Part model, mm, in its own coordinate system. A direction names the side the tool comes from. Round coordinates to 2 decimals unless told otherwise and drop trailing zeros. Loops run counter-clockwise (first coordinate to the right, second up) from the corner with the lowest first, then second, coordinate; pieces in that order, holes last. Notation, with made-up numbers: M 44.5,-20.75 L 80.5,-20.75 A21 ccw 80.5,10.25 Z; hole C 83.5,-15.5 d5. An arc over 180 degrees is marked long. Put each result on its own line as item: value. Start each with the question number.
1) Slice it at A-A on x = 0. Give the cut face in (y, z).
2) Pull direction Z, two halves, no side cores. Call faces 6 (the flat face through (0, 0, -22.149)), 7 (the flat face through (9.112, 0, -11)), 8 (the cylindrical face through (-27.2, 0, -10.4)): +Z half, -Z half, draft (parallel to the pull), parting line (faces both ways), or undercut.
3) Drop flat-ended pins along their axis: pin 1 Ø6 at (y, z) = (0.5, -15.5) entering from -X; pin 2 Ø6 at (x, z) = (-32, -2) entering from +Y; pin 3 Ø1.5 at (x, z) = (-21, -12) entering from +Y; pin 4 Ø6 at (y, z) = (17.5, -3) entering from +X. Give the stop position or say it passes through.
4) Slice it at C-C on y = -19. Give the cut face in (x, z).
5) Slice it at B-B on z = -1. Give the cut face in (x, y).
6) Probe line 1 along X through (y, z) = (-7, 6); line 2 along X through (y, z) = (-5, 16); line 3 along Y through (x, z) = (-37.5, 21.9). List the from-to ranges inside material, lowest first.
7) Slice it at D-D on x = -17. Give the cut face in (y, z), then the cut area to 3 significant figures.
8) Which spindle directions (+Z, -Z, +X, -X, +Y, -Y) get a long thin tool onto all of the face, cutting with end or side? Do faces 1 (the flat face through (29, -2.75, -9)), 2 (the flat face through (0, 2.75, -9)), 3 (the cylindrical face through (-1.84, 14.04, 33.52)), 4 (the flat face through (20.098, 0, -11)), 5 (the flat face through (-38.322, 0, -11)). Say none if no direction does.
```python
from build123d import *

# Parameters (mm, degrees)
SKETCH1_R                = 14.1605
BOSS_EXTRUDE1_DEPTH      = 43.18
SKETCH3_W                = 18.2245
SKETCH3_H                = 22.1488
SKETCH3_R                = 4.2545
BOSS_EXTRUDE2_DEPTH      = 2.74955
BOSS_EXTRUDE2_DEPTH_BACK = 2.74955
LPATTERN1_COUNT          = 2
LPATTERN1_PITCH          = 29.21
LPATTERN1_2_COUNT        = 2
LPATTERN1_2_PITCH        = 29.21
BOSS_EXTRUDE3_START      = 20.32
SKETCH4_R                = 3.048
BOSS_EXTRUDE3_DEPTH      = 3.81
BOSS_EXTRUDE4_START      = -30.48
BOSS_EXTRUDE4_DEPTH      = 2.54


with BuildPart() as part:
    # Sketch1 → Boss-Extrude1 (new body)
    with BuildSketch(Plane.XY):
        Circle(SKETCH1_R)
    extrude(amount=BOSS_EXTRUDE1_DEPTH)

    # Sketch3 → Boss-Extrude2 (add, two sides)
    with BuildSketch(Plane(origin=(0, 0, 0), x_dir=(1, 0, 0), z_dir=(0, 1, 0))) as boss_extrude2_sk:
        with Locations((0, 11.0744)):
            Rectangle(SKETCH3_W, SKETCH3_H)
        with Locations((0, 14.1478)):
            Circle(SKETCH3_R, mode=Mode.SUBTRACT)
    extrude(amount=BOSS_EXTRUDE2_DEPTH)
    extrude(boss_extrude2_sk.sketch, amount=-BOSS_EXTRUDE2_DEPTH_BACK)


with BuildPart() as lpattern1_1:
    # LPattern1: pattern copy
    add(part.part.moved(Location(Vector(1, 0, 0) * (1 * LPATTERN1_PITCH))))


with BuildPart() as lpattern1_2_1:
    # LPattern1 2: pattern copy
    add(part.part.moved(Location(Vector(-1, 0, 0) * (1 * LPATTERN1_2_PITCH))))


with BuildPart() as lpattern1_2_2:
    # LPattern1 2: pattern copy
    add(lpattern1_1.part.moved(Location(Vector(-1, 0, 0) * (1 * LPATTERN1_2_PITCH))))


with BuildPart() as part_1:
    add(part.part)

    add(lpattern1_1.part)  # Boss-Extrude3 merges LPattern1_1

    add(lpattern1_2_1.part)  # Boss-Extrude3 merges LPattern1 2_1

    add(lpattern1_2_2.part)  # Boss-Extrude3 merges LPattern1 2_2
    # Sketch4 → Boss-Extrude3 (add)
    with BuildSketch(Plane.XY.offset(BOSS_EXTRUDE3_START)):
        with BuildLine():
            Line((-37.5, 24), (37.5, 24))
            ThreePointArc((37.5, 24), (44.571067812, 21.071067812), (47.5, 14))
            Line((47.5, 14), (47.5, -14))
            ThreePointArc((47.5, -14), (44.571067812, -21.071067812), (37.5, -24))
            Line((37.5, -24), (-37.5, -24))
            ThreePointArc((-37.5, -24), (-44.571067812, -21.071067812), (-47.5, -14))
            Line((-47.5, -14), (-47.5, 14))
            ThreePointArc((-47.5, 14), (-44.571067812, 21.071067812), (-37.5, 24))
        make_face()
        with Locations((-37.5, 19)):
            Circle(SKETCH4_R, mode=Mode.SUBTRACT)
        with Locations((37.5, 19)):
            Circle(SKETCH4_R, mode=Mode.SUBTRACT)
        with Locations((37.5, -19)):
            Circle(SKETCH4_R, mode=Mode.SUBTRACT)
        with Locations((-37.5, -19)):
            Circle(SKETCH4_R, mode=Mode.SUBTRACT)
    extrude(amount=BOSS_EXTRUDE3_DEPTH)

    # Sketch6 → Boss-Extrude4 (add)
    with BuildSketch(Plane.XY.offset(43.18).offset(BOSS_EXTRUDE4_START)):
        with BuildLine():
            Line((-1.27, 14.103434342), (-1.27, 15.119434342))
            Line((-1.27, 15.119434342), (1.27, 15.119434342))
            Line((1.27, 15.119434342), (1.27, 14.103434342))
            ThreePointArc((1.27, 14.103434342), (0, 14.1605), (-1.27, 14.103434342))
        make_face()
    extrude(amount=-BOSS_EXTRUDE4_DEPTH)


solid = part_1.part
```
Recorded:
1. outline: M -24,20.32 L -14.16,20.32 L -14.16,0 L -2.75,0 L -2.75,-9.89 L 2.75,-9.89 L 2.75,0 L 14.16,0 L 14.16,10.16 L 15.12,10.16 L 15.12,12.7 L 14.16,12.7 L 14.16,20.32 L 24,20.32 L 24,24.13 L 14.16,24.13 L 14.16,43.18 L -14.16,43.18 L -14.16,24.13 L -24,24.13 Z; M -2.75,-22.15 L 2.75,-22.15 L 2.75,-18.4 L -2.75,-18.4 Z
2. face 6: -Z half
2. face 7: draft
2. face 8: undercut
3. pin 1: stops at x = -38.32
3. pin 2: stops at y = 14.15
3. pin 3: stops at y = 2.75
3. pin 4: passes through
4. outline: M -46.16,20.32 L -40.55,20.32 L -40.55,24.13 L -46.16,24.13 Z; M -34.45,20.32 L 34.45,20.32 L 34.45,24.13 L -34.45,24.13 Z; M 40.55,20.32 L 46.16,20.32 L 46.16,24.13 L 40.55,24.13 Z
5. outline: M -38.32,-2.75 L -20.1,-2.75 L -20.1,2.75 L -38.32,2.75 Z; M -9.11,-2.75 L 9.11,-2.75 L 9.11,2.75 L -9.11,2.75 Z; M 20.1,-2.75 L 38.32,-2.75 L 38.32,2.75 L 20.1,2.75 Z
6. line 1: x = -41.52 to -16.9, -12.31 to 12.31, 16.9 to 41.52
6. line 2: x = -42.46 to -15.96, -13.25 to 13.25, 15.96 to 42.46
6. line 3: y = -24 to -22.05, -15.95 to 15.95, 22.05 to 24
7. outline: M -24,20.32 L -7.17,20.32 L -7.17,0 L 7.17,0 L 7.17,20.32 L 24,20.32 L 24,24.13 L 7.17,24.13 L 7.17,43.18 L -7.17,43.18 L -7.17,24.13 L -24,24.13 Z
7. area: 748 mm2
8. face 1: -Z, +X, -X, -Y
8. face 2: -Z, +X, -X, +Y
8. face 3: +Z
8. face 4: -Z, +Y, -Y
8. face 5: -Z, -X, +Y, -Y
